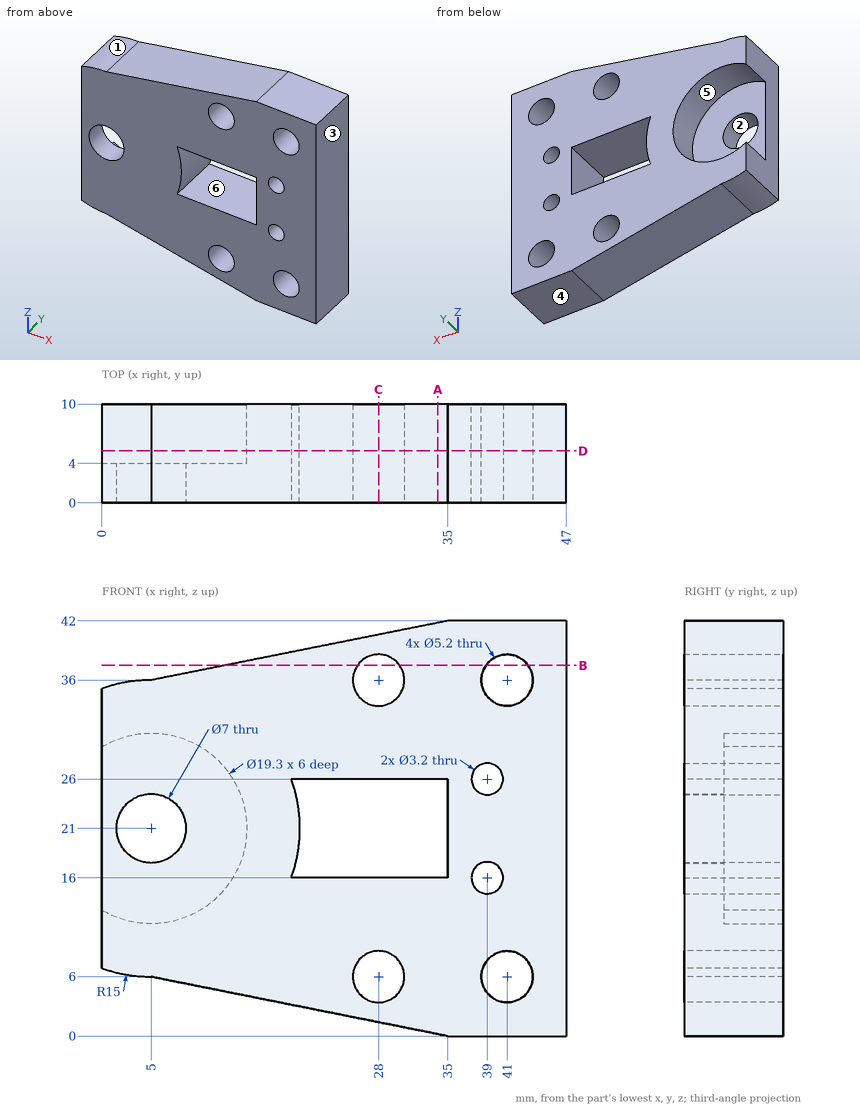
Geometry: see drawing. Coordinates: mm, zero at the bounding-box minimum. A direction names the side the tool comes from. Round coordinates to 2 decimals unless told otherwise and drop trailing zeros. Order: outer loops, then holes, each group sorted by start corner. A loop starts at its lowest first (then second) coordinate and runs counter-clockwise, first axis right, second up. Notation, with made-up numbers: (84, -11.5) - (106, -11.5) arc R19 cw to (106, -5.5) - close; hole circle Ø11 at (-17.75, 69). An arc over 180 degrees is marked (long way). Use a Markdown table: item, result. Add a question column.
1. Line query: probe 1 along Z at (x, y) = (41, 7.5); probe 2 along Z at (x, y) = (39, 7.25); probe 3 along X at (y, z) = (6.65, 21). Output: solid intervals per line, ascending.
2. First-contact query: pin 1 (1.5 mm diameter, centred on x = 28, y = 8.5, fed in from -Z); pin 2 (4 mm diameter, centred on x = 41, z = 6, fed in from +Y); pin 3 (3 mm diameter, centred on y = 4.5, z = 21, fed in from -X); pin 4 (6 mm diameter, centred on x = 16.5, y = 8.5, fed in from -Z). Flat tips, straight axial feed; report the tip coordinate or a pass-through.
3. Section query C-C (x = 28). Return the cut outline in (y, z), then the cut area to 3 significant figures.
4. Section query B-B (z = 37.5). Return the cut outline in (x, y), then the cut area to 3 significant figures.
5. Section query D-D (y = 5.25). Return the cut outline in (x, z), then the cut area to 3 significant figures.
6. Set-up query: the marked faces 4, 5 and 6. Return all of +Z, -Z, +X, -X, +Y, -Y with unobstructed straight access to the full face (end or side cutting, diameter ignored); none if empty.
7. Section query A-A (x = 34). Return the cut outline in (y, z).
8. Mould query, pull axis Z, two halves, no side actions, for the marked faces 1, 2 and 3. Classes: +Z half, -Z half, draft (parallel to the pull), parting line (faces both ways), or undercut.
Derived:
| question | item | result |
|---|---|---|
| 1 | probe 1 | 0 to 3.4, 8.6 to 33.4, 38.6 to 42 |
| 1 | probe 2 | 0 to 4.34, 7.66 to 14.4, 17.6 to 24.4, 27.6 to 34.34, 37.66 to 42 |
| 1 | probe 3 | 14.65 to 20, 35 to 47 |
| 2 | pin 1 | z = 1.25 |
| 2 | pin 2 | through |
| 2 | pin 3 | x = 0 |
| 2 | pin 4 | z = 3.1 |
| 3 | outline | (0, 1.4) - (10, 1.4) - (10, 3.4) - (0, 3.4) - close; (0, 8.6) - (10, 8.6) - (10, 16) - (0, 16) - close; (0, 26) - (10, 26) - (10, 33.4) - (0, 33.4) - close; (0, 38.6) - (10, 38.6) - (10, 40.6) - (0, 40.6) - close |
| 3 | area | 188 mm2 |
| 4 | outline | (12.5, 0) - (25.88, 0) - (25.88, 10) - (12.5, 10) - close; (30.12, 0) - (38.88, 0) - (38.88, 10) - (30.12, 10) - close; (43.12, 0) - (47, 0) - (47, 10) - (43.12, 10) - close |
| 4 | area | 260 mm2 |
| 5 | outline | (0, 6.86) arc R15 ccw to (5, 6) - (35, 0) - (47, 0) - (47, 42) - (35, 42) - (5, 36) arc R15 ccw to (0, 35.14) - (0, 29.25) arc R9.65 cw (long way) to (0, 12.75) - close; hole (19.14, 16) - (35, 16) - (35, 26) - (19.14, 26) arc R15 cw to start; hole circle Ø5.2 at (28, 6); hole circle Ø5.2 at (28, 36); hole circle Ø3.2 at (39, 16); hole circle Ø3.2 at (39, 26); hole circle Ø5.2 at (41, 6); hole circle Ø5.2 at (41, 36) |
| 5 | area | 1,240 mm2 |
| 6 | face 4 | -Z, +X, -X, +Y, -Y |
| 6 | face 5 | +Y |
| 6 | face 6 | +Y, -Y |
| 7 | outline | (0, 0.2) - (10, 0.2) - (10, 16) - (0, 16) - close; (0, 26) - (10, 26) - (10, 41.8) - (0, 41.8) - close |
| 8 | face 1 | +Z half |
| 8 | face 2 | undercut |
| 8 | face 3 | draft |
